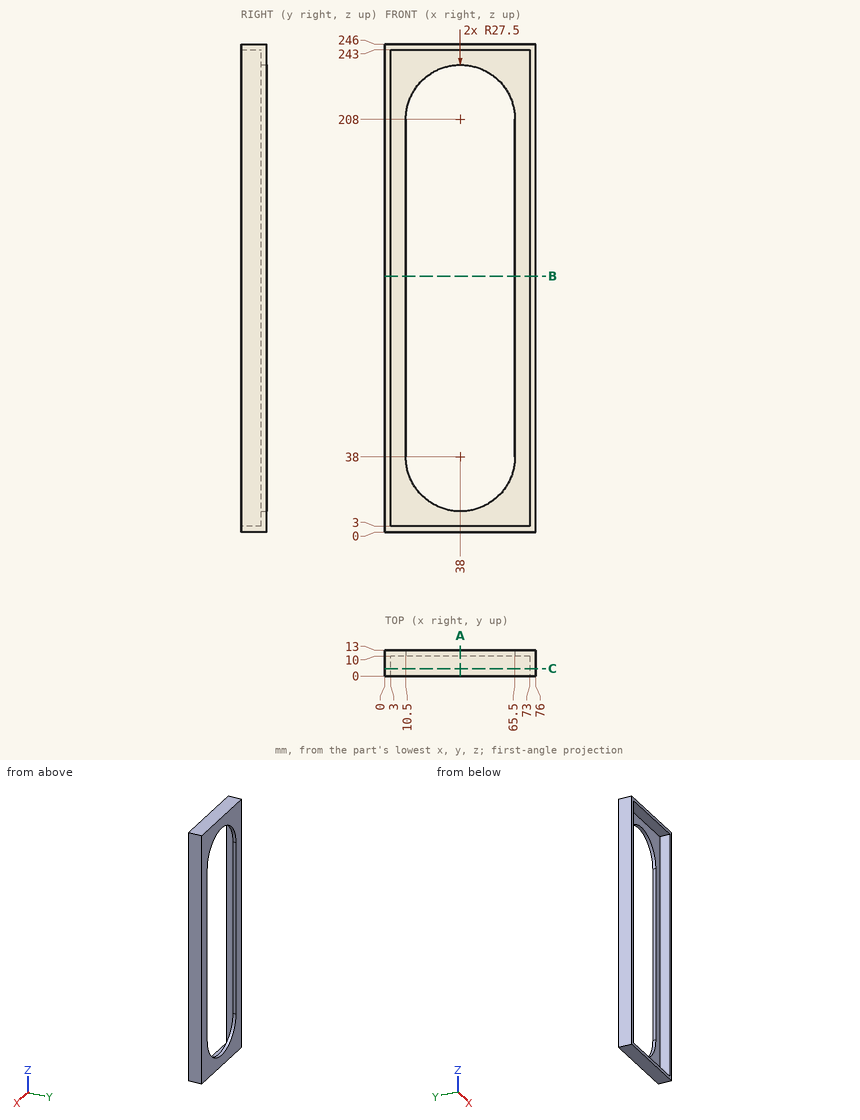
Could you check a few things on this drawing? It's one solid part, dimensions in mm from its lowest x, y, z. Give positions to 0.01 mm unless a question says otherwise; leave off trailing zeros. Order: outer loops, then holes, each group sorted by start corner. A loop starts at its lowest first (then second) coordinate and runs counter-clockwise, first axis right, second up. Notation, with made-up numbers: (15.5, -40) -> (27.5, -40) arc R12 ccw to (27.5, -24) -> close; hole circle Ø6 at (-30.75, -18). An arc over 180 degrees is marked (long way). Answer in a Markdown table with one row per item. Add a question column.
Item 1: I'm going to push flat-ended pins straight in: P1, Ø5, axis at y = 3.5, z = 75.5, coming from the -X side; P2, Ø4, axis at x = 68, z = 194.5, coming from the -Y side. Where does each tip first touch, or does it pass through?
Item 2: Imagine slicing it at A-A (x = 38). List the corners of the cut face in (y, z) for me.
Item 3: Imagine slicing it at B-B (z = 129). List the corners of the cut face in (x, y) for me.
Item 4: Please list where these lines run through material, in increasing order: probe 1 along X at (y, z) = (4.5, 12.5); probe 2 along Z at (x, y) = (31, 5); probe 3 along X at (y, z) = (12.75, 123.5).
Item 5: Imagine slicing it at C-C (y = 3.75). List the corners of the cut face in (x, z) for me, and give its area (3 significant figures).
Result:
| question | item | result |
|---|---|---|
| 1 | P1 | x = 0 |
| 1 | P2 | y = 10 |
| 2 | outline | (0, 0) -> (13, 0) -> (13, 10.5) -> (10, 10.5) -> (10, 3) -> (0, 3) -> close; (0, 243) -> (10, 243) -> (10, 235.5) -> (13, 235.5) -> (13, 246) -> (0, 246) -> close |
| 3 | outline | (0, 0) -> (3, 0) -> (3, 10) -> (10.5, 10) -> (10.5, 13) -> (0, 13) -> close; (65.5, 10) -> (73, 10) -> (73, 0) -> (76, 0) -> (76, 13) -> (65.5, 13) -> close |
| 4 | probe 1 | 0 to 3, 73 to 76 |
| 4 | probe 2 | 0 to 3, 243 to 246 |
| 4 | probe 3 | 0 to 10.5, 65.5 to 76 |
| 5 | outline | (0, 0) -> (76, 0) -> (76, 246) -> (0, 246) -> close; hole (3, 3) -> (73, 3) -> (73, 243) -> (3, 243) -> close |
| 5 | area | 1,900 mm2 |
